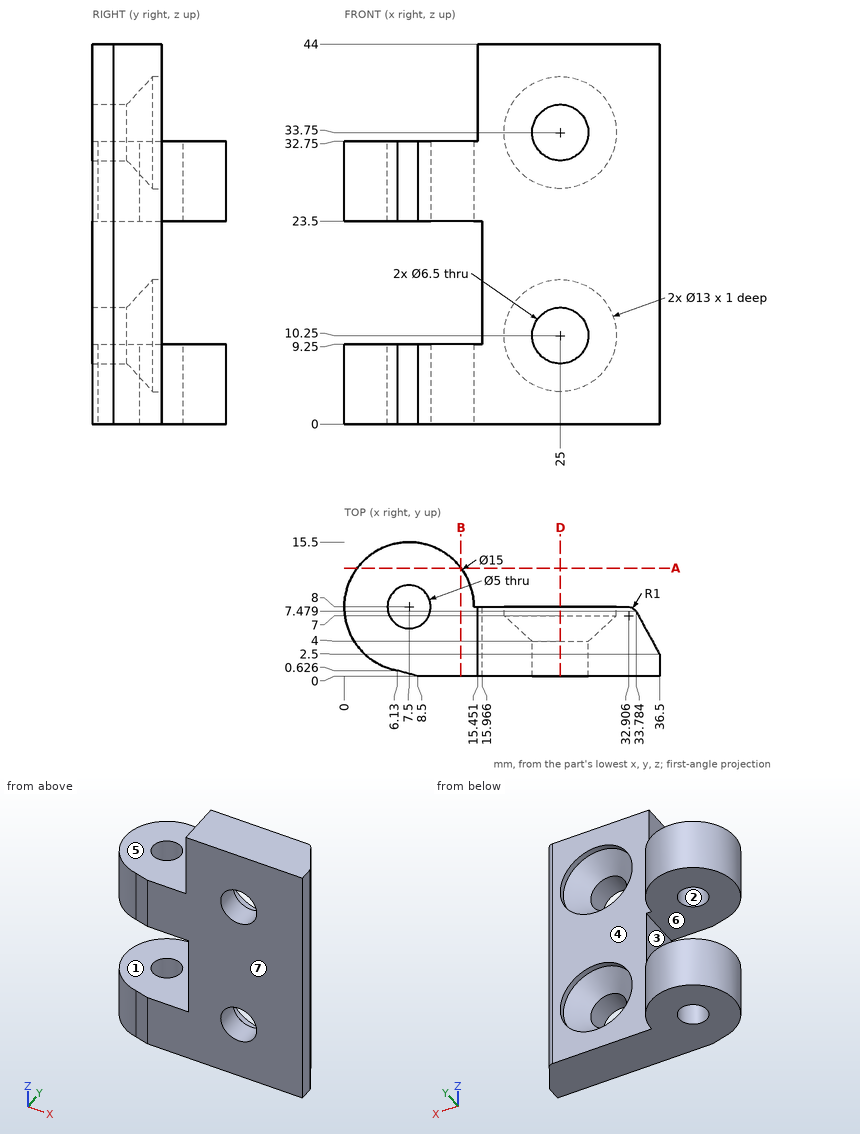
Print and shaded views of the part. All mm, measured from the part's lowest x, y and z. A direction names the side the tool comes from. Coordinates: 2 decimals unless noted, no trailing zeros. Order: outer loops, then holes, each group sorted by start corner. A loop starts at its lowest first (then second) coordinate and runs counter-clockwise, first axis right, second up. Notation, with made-up numbers: (58.25, -19.75) -> (62.25, -19.75) arc R24 ccw to (62.25, 2.25) -> close; hole circle Ø5 at (5.25, 44). An arc over 180 degrees is marked (long way). Answer as a JSON object with one key per item and string values. Group by question number.
1) Cut at D-D, the plane x = 25. Write the cut outline in (y, z).
2) Which spindle directions (+Z, -Z, +X, -X, +Y, -Y) get a long thin tool onto all of the face, cutting with end or side? Do the marked faces 4, 5, 6 and 7. Say none if no direction does.
3) Cut at A-A, the plane y = 12.5. Write the cut outline in (x, z), then the cut area to 3 significant figures.
4) Pull direction X, two halves, no side cores. Call the marked faces 1, 2 and 3: +X half, -X half, draft (parallel to the pull), parting line (faces both ways), or undercut.
5) Cut at B-B, the plane x = 13.5. Write the cut outline in (y, z).
6) Drill centre lines: L1, parallel to Z at x = 5, y = 10.5; L2, parallel to Y at x = 7.5, z = 27.5 (1 decimal); L3, parallel to Y at x = 17, z = 34.5. Where is each one in solid material? Low to high.
7) Flat gauge pins, fed straight in: pin 1 (1.5 mm diameter, centred on x = 17.5, z = 32.5, fed in from +Y); pin 2 (1 mm diameter, centred on x = 8, y = 12, fed in from +Z); pin 3 (9 mm diameter, centred on y = 3.5, z = 40.5, fed in from -X); pin 4 (4.5 mm diameter, centred on x = 7.5, y = 8, fed in from -Z). Where does each tip first touch, or does it go through?
Check values:
{
 "1": {"outline": "(0, 0) -> (8, 0) -> (8, 3.75) -> (7, 3.75) -> (4, 7) -> (0, 7) -> close; (0, 13.5) -> (4, 13.5) -> (7, 16.75) -> (8, 16.75) -> (8, 27.25) -> (7, 27.25) -> (4, 30.5) -> (0, 30.5) -> close; (0, 37) -> (4, 37) -> (7, 40.25) -> (8, 40.25) -> (8, 44) -> (0, 44) -> close"},
 "2": {"face 4": "+Z, -Z, +X, +Y", "face 5": "+Z, -X, +Y, -Y", "face 6": "-X, +Y, -Y", "face 7": "+Z, -Z, +X, -X, -Y"},
 "3": {"outline": "(1.5, 0) -> (13.5, 0) -> (13.5, 9.25) -> (1.5, 9.25) -> close; (1.5, 23.5) -> (13.5, 23.5) -> (13.5, 32.75) -> (1.5, 32.75) -> close", "area": "222 mm²"},
 "4": {"face 1": "draft", "face 2": "undercut", "face 3": "-X half"},
 "5": {"outline": "(0, 0) -> (12.5, 0) -> (12.5, 9.25) -> (0, 9.25) -> close; (0, 23.5) -> (12.5, 23.5) -> (12.5, 32.75) -> (0, 32.75) -> close"},
 "6": {"L1": "z = 0 to 9.25, 23.5 to 32.75", "L2": "y = 0.3 to 5.5, 10.5 to 15.5", "L3": "y = 0 to 8"},
 "7": {"pin 1": "stops at y = 8", "pin 2": "stops at z = 32.75", "pin 3": "stops at x = 15.45", "pin 4": "passes through"}
}
